```python
from build123d import *

# Parameters (mm, degrees)
SKETCH_1_R          = 1.00000054
SKETCH_1_W          = 13
SKETCH_1_H          = 12
SKETCH_1_W_2        = 35.054000855
SKETCH_1_H_2        = 47
SKETCH_1_W_3        = 4
SKETCH_1_H_3        = 22
EXTRUDE_1_DEPTH     = 2
FILLET_2_R          = 3
SKETCH_2_R          = 1.5
CUT_EXTRUDE_1_DEPTH = 120.290710997


with BuildPart() as part:
    # 草图1 → 凸台-拉伸1 (new body)
    # profile 1 of 2: a face of its own
    with BuildSketch(Plane.XY.offset(11.133645354)):
        Polygon((86.391138075, 82.236518604), (36.391138075, 82.236518604), (36.391138075, -7.763481396), (86.391138075, -7.763481396), (86.391138075, 4.236518604), (73.391138075, 4.236518604), (73.391138075, 18.736518604), (86.391138075, 18.736518604), align=None)
        with Locations((46.291138075, -0.363481396)):
            Circle(SKETCH_1_R, mode=Mode.SUBTRACT)
        with Locations((45.891138075, 24.236518604)):
            Circle(SKETCH_1_R, mode=Mode.SUBTRACT)
        with Locations((61.391138075, 10.236518604)):
            Rectangle(SKETCH_1_W, SKETCH_1_H, mode=Mode.SUBTRACT)
        with Locations((76.491138075, -0.363481396)):
            Circle(SKETCH_1_R, mode=Mode.SUBTRACT)
        with Locations((76.891138075, 24.236518604)):
            Circle(SKETCH_1_R, mode=Mode.SUBTRACT)
        with Locations((61.385138076, 49.650651887)):
            Rectangle(SKETCH_1_W_2, SKETCH_1_H_2, mode=Mode.SUBTRACT)
        with Locations((45.891138075, 75.236518604)):
            Circle(SKETCH_1_R, mode=Mode.SUBTRACT)
        with Locations((82.391138075, 37.236518604)):
            Rectangle(SKETCH_1_W_3, SKETCH_1_H_3, mode=Mode.SUBTRACT)
        with Locations((76.891138075, 75.236518604)):
            Circle(SKETCH_1_R, mode=Mode.SUBTRACT)
    # profile 2 of 2: a face of its own
    with BuildSketch(Plane.XY.offset(11.133645354)):
        with Locations((61.385138076, 49.650651887)):
            Rectangle(SKETCH_1_W_2, SKETCH_1_H_2)
    extrude(amount=EXTRUDE_1_DEPTH)

    # 圆角2
    fillet_2_edges = [part.edges().sort_by_distance(p)[0] for p in [
        (86.391138075, 4.236518604, 12.133645354),
        (86.391138075, -7.763481396, 12.133645354),
        (36.391138075, -7.763481396, 12.133645354),
        (36.391138075, 82.236518604, 12.133645354),
        (86.391138075, 82.236518604, 12.133645354),
        (86.391138075, 18.736518604, 12.133645354),
    ]]
    fillet(fillet_2_edges, radius=FILLET_2_R)

    # 草图2 → 切除-拉伸1 (cut, through all)
    with BuildSketch(Plane.XY.offset(13.133645354)):
        with Locations((40.391138075, 78.236518604)):
            Circle(SKETCH_2_R)
        with Locations(Location((82.391138075, 78.236518604, 0), (0, 0, 180))):
            Circle(SKETCH_2_R)
        with Locations((40.391138075, 23.236518604)):
            Circle(SKETCH_2_R)
        with Locations(Location((82.391138075, 23.236518604, 0), (0, 0, 180))):
            Circle(SKETCH_2_R)
        with Locations(Location((40.391138075, 51.236518604, 0), (0, 0, 180))):
            Circle(SKETCH_2_R)
        with Locations((82.391138075, 51.236518604)):
            Circle(SKETCH_2_R)
        with Locations((82.391138075, -3.763481396)):
            Circle(SKETCH_2_R)
        with Locations(Location((40.391138075, -3.763481396, 0), (0, 0, 180))):
            Circle(SKETCH_2_R)
    extrude(amount=-CUT_EXTRUDE_1_DEPTH, mode=Mode.SUBTRACT)


solid = part.part
```
Model file for the job. Use its own axes, mm. A direction names the side the tool comes from. Coordinates: 2 decimals unless noted, no trailing zeros. Write each loop counter-clockwise with the first axis right and the second up, starting at its lowest first coordinate (ties: lowest second). Pieces come first, ordered by that corner, then holes. Notation, with made-up numbers: (56, 16) - (100, 16) arc R15 ccw to (100, 24) - close; hole circle Ø9 at (-8, 24.5). An arc over 180 degrees is marked (long way). One line per item, written item: value. Start each with the question number.
1. Slice it at A-A (y = 37). Write the cut outline in (x, z), plus the area to 3 significant figures.
2. Probe line 1 (X direction, y = 36, z = 11.4); line 2 (X direction, y = 24.5, z = 12.35); line 3 (Y direction, x = 84, z = 12). List the from-to ranges inside material, lowest first. Write a range as from..to.
3. Slice it at B-B (x = 40.5). Write the cut outline in (y, z).
4. Mould opens along Y. For faces 1 (the cylindrical face through (37.29, 81.38, 12.15)), 2 (the flat face through (61, 16.237, 12)), 3 (the flat face through (61, -7.763, 12)) say: released by +Y, released by -Y, zero draft, split by the parting line, or undercut.
5. Tool access for faces 4 (the flat face through (78, 18.737, 12)), 5 (the flat face through (82, 48.237, 12)), 6 (the flat face through (61, 38, 13.134)): list every direction of +Z, -Z, +X, -X, +Y, -Y with a clear straight run to the whole face (end or side of a thin tool).
6. Slice it at C-C (z = 12.35). Count the separate pieces of the cut face and the enclosed holes in it, plus the area to 3 significant figures.
Answers below:
1. outline: (36.39, 11.13) - (80.39, 11.13) - (80.39, 13.13) - (36.39, 13.13) - close; (84.39, 11.13) - (86.39, 11.13) - (86.39, 13.13) - (84.39, 13.13) - close
1. area: 92.0 mm^2
2. line 1: x = 36.39..80.39, 84.39..86.39
2. line 2: x = 36.39..39.58, 41.2..44.93, 46.86..75.93, 77.86..81.58, 83.2..86.39
2. line 3: y = -7.7..4.17, 18.8..26.24, 48.24..82.17
3. outline: (-7.76, 11.13) - (-5.26, 11.13) - (-5.26, 13.13) - (-7.76, 13.13) - close; (-2.27, 11.13) - (21.74, 11.13) - (21.74, 13.13) - (-2.27, 13.13) - close; (24.73, 11.13) - (49.74, 11.13) - (49.74, 13.13) - (24.73, 13.13) - close; (52.73, 11.13) - (76.74, 11.13) - (76.74, 13.13) - (52.73, 13.13) - close; (79.73, 11.13) - (82.24, 11.13) - (82.24, 13.13) - (79.73, 13.13) - close
4. face 1: released by +Y
4. face 2: undercut
4. face 3: released by -Y
5. face 4: +Z, -Z, +X
5. face 5: +Z, -Z
5. face 6: +Z, +X, -X, +Y, -Y
6. separate pieces: 1
6. enclosed holes: 16
6. area: 3,980 mm^2
